from build123d import *

# Parameters (mm, degrees)
F2_SIZE  = 1
F3_R     = 5
F4_DEPTH = 60.001


with BuildPart() as f1:
    # F0 (on Front) → F1 (revolve)
    with BuildSketch(Plane.XZ):
        Polygon((-45.251393, 20), (-45.251393, 0), (14.748607, 0), (14.748607, 15), (-25.251393, 15), (-25.251393, 20), align=None)
    revolve(axis=Axis((-14.02186, 0, 0), (1, 0, 0)))

    # F2
    f2_edges = [f1.edges().sort_by_distance(p)[0] for p in [
        (14.748607, 0, -15),
    ]]
    chamfer(f2_edges, length=F2_SIZE)

    # F3 (on face) → F4 (cut, through all)
    with BuildSketch(Plane.YZ.offset(14.748607)):
        Circle(F3_R)
    extrude(amount=-F4_DEPTH, mode=Mode.SUBTRACT)


solid = f1.part
Here's how the part is built. I have some questions about the finished solid (model axes, mm). Coordinates: 2 decimals unless noted, no trailing zeros. Write each loop counter-clockwise with the first axis right and the second up, starting at its lowest first coordinate (ties: lowest second). Pieces come first, ordered by that corner, then holes. Notation, with made-up numbers: (34, -16.5) - (93, -16.5) arc R16 cw to (93, 12.5) - close; hole circle Ø9 at (12.25, 67). An arc over 180 degrees is marked (long way). Use one line per item in the form item = value.
1) Suppose I cut it at A-A, the plane y = 0. Write out the boundary of the cut face in (x, z).
Solved:
outline = (-45.25, -20) - (-25.25, -20) - (-25.25, -15) - (13.75, -15) - (14.75, -14) - (14.75, -5) - (-45.25, -5) - close; (-45.25, 5) - (14.75, 5) - (14.75, 14) - (13.75, 15) - (-25.25, 15) - (-25.25, 20) - (-45.25, 20) - close
2) I'm going to push flat-ended pins straight in: P1, Ø3, axis at x = -5, y = 10.5, coming from the -Z side; P2, Ø2, axis at x = -21, y = 11, coming from the +Z side; P3, Ø1.5, axis at x = -34, y = -14.5, coming from the +Z side. Where does each tip first touch, or does it pass through?
Solved:
P1 = -12
P2 = 11.18
P3 = 14.52
3) Thinking about a two-plate mould opening in Y: for faces 1 (the cylindrical face through (-6.024, -0.66, -14.985)), 2 (the flat face through (-25.251, -15, -3)), 3 (the cylindrical face through (-14.83, -1.08, -4.88)), which applies, released by +Y, released by -Y, zero draft, split by the parting line, or undercut?
Solved:
face_1 = split by the parting line
face_2 = zero draft
face_3 = undercut
4) I need wall thicknesses on line 1 (Z direction, x = -11, y = 0); line 2 (Z direction, x = -29, y = 0); line 3 (Y direction, x = -37.5, z = 2). Which ranges of each line are inside material? Lowest first, please.
Solved:
line_1 = -15 to -5, 5 to 15
line_2 = -20 to -5, 5 to 20
line_3 = -19.9 to -4.58, 4.58 to 19.9
